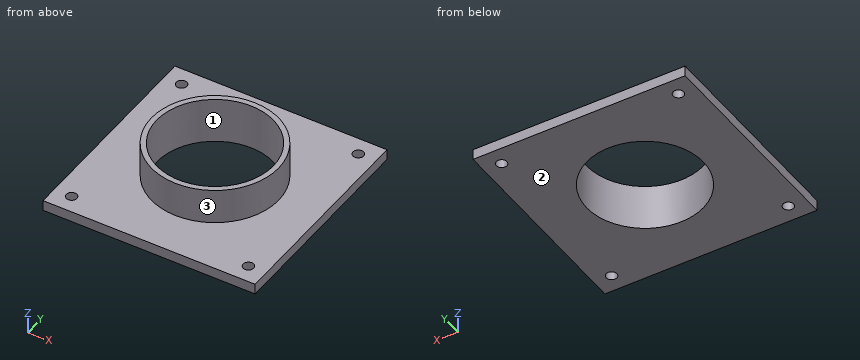
from build123d import *

# Parameters (mm, degrees)
SKETCH1_W           = 60
SKETCH1_H           = 60
SKETCH1_R           = 16.5
SKETCH1_R_2         = 1.5
BOSS_EXTRUDE1_DEPTH = 3
SKETCH2_R           = 18
SKETCH2_R_2         = 16.5
BOSS_EXTRUDE2_DEPTH = 10


with BuildPart() as part:
    # Sketch1 → Boss-Extrude1 (new body)
    with BuildSketch(Plane.XY):
        with Locations((30, 30)):
            Rectangle(SKETCH1_W, SKETCH1_H)
        with Locations((30, 30)):
            Circle(SKETCH1_R, mode=Mode.SUBTRACT)
        with Locations((5, 55)):
            Circle(SKETCH1_R_2, mode=Mode.SUBTRACT)
        with Locations(Location((55, 55, 0), (0, 0, 180))):
            Circle(SKETCH1_R_2, mode=Mode.SUBTRACT)
        with Locations((55, 5)):
            Circle(SKETCH1_R_2, mode=Mode.SUBTRACT)
        with Locations(Location((5, 5, 0), (0, 0, 180))):
            Circle(SKETCH1_R_2, mode=Mode.SUBTRACT)
    extrude(amount=BOSS_EXTRUDE1_DEPTH)

    # Sketch2 → Boss-Extrude2 (add)
    with BuildSketch(Plane.XY.offset(3)):
        with Locations((30, 30)):
            Circle(SKETCH2_R)
        with Locations((30, 30)):
            Circle(SKETCH2_R_2, mode=Mode.SUBTRACT)
    extrude(amount=BOSS_EXTRUDE2_DEPTH)


solid = part.part
Can you work these out from the model? Positions are in its coordinate system, mm. Face numbers are marked on the shaded views. Give positions to 0.01 mm unless a question says otherwise; leave off trailing zeros. Loops run counter-clockwise (first coordinate to the right, second up) from the corner with the lowest first, then second, coordinate; pieces in that order, holes last. Notation, with made-up numbers: (71, 84) -> (112, 84) arc R33 ccw to (112, 118) -> close; hole circle Ø10 at (45, -11). An arc over 180 degrees is marked (long way). Write item = value, one per line.
1) Suppose I cut it at C-C on x = 21.5. Write out the boundary of the cut face in (y, z).
Check result:
outline = (0, 0) -> (15.86, 0) -> (15.86, 13) -> (14.13, 13) -> (14.13, 3) -> (0, 3) -> close; (44.14, 0) -> (60, 0) -> (60, 3) -> (45.87, 3) -> (45.87, 13) -> (44.14, 13) -> close
2) Will these pins go through, and if not, where does the flat tip stop? pin 1 (2 mm diameter, centred on y = 24.5, z = 11, fed in from +X); pin 2 (6 mm diameter, centred on x = 36.5, y = 40, fed in from +Z); pin 3 (2 mm diameter, centred on y = 19.5, z = 8.5, fed in from -X); pin 4 (3.5 mm diameter, centred on x = 55, y = 5, fed in from +Z).
Check result:
pin_1 = 47.43
pin_2 = through
pin_3 = 14.71
pin_4 = 3
3) Thinking about a two-plate mould opening in Y: for the marked faces 1, 2 and 3, which applies, released by +Y, released by -Y, zero draft, split by the parting line, or undercut?
Check result:
face_1 = undercut
face_2 = zero draft
face_3 = split by the parting line
4) Suppose I cut it at A-A on y = 30. Write out the boundary of the cut face in (x, z), then the cut area to 3 significant figures.
Check result:
outline = (0, 0) -> (13.5, 0) -> (13.5, 13) -> (12, 13) -> (12, 3) -> (0, 3) -> close; (46.5, 0) -> (60, 0) -> (60, 3) -> (48, 3) -> (48, 13) -> (46.5, 13) -> close
area = 111 mm2
5) Suppose I cut it at B-B on x = 5. Write out the boundary of the cut face in (y, z), then the cut area to 3 significant figures.
Check result:
outline = (0, 0) -> (3.5, 0) -> (3.5, 3) -> (0, 3) -> close; (6.5, 0) -> (53.5, 0) -> (53.5, 3) -> (6.5, 3) -> close; (56.5, 0) -> (60, 0) -> (60, 3) -> (56.5, 3) -> close
area = 162 mm2
6) I need wall thicknesses on L1, parallel to Y at x = 55, z = 2.3; L2, parallel to Z at x = 4, y = 19.5; L3, parallel to X at y = 38, z = 2. Which ranges of each line are inside material? Lowest first, please. Write a range as from..to.
Check result:
L1 = 0..3.5, 6.5..53.5, 56.5..60
L2 = 0..3
L3 = 0..15.57, 44.43..60
